Source: CAD feature listing. Evaluate the final solid. Frame: model axes, mm. Face numbers are marked on the shaded views. A direction names the side the tool comes from. Give positions to 0.01 mm unless a question says otherwise; leave off trailing zeros. Order: outer loops, then holes, each group sorted by start corner. A loop starts at its lowest first (then second) coordinate and runs counter-clockwise, first axis right, second up. Notation, with made-up numbers: (-1.5, 74.25) - (2.5, 74.25) arc R24 cw to (2.5, 92.25) - close; hole circle Ø7 at (9, 35). An arc over 180 degrees is marked (long way). Answer as CSV lines item,"result".
```python
from build123d import *

# Parameters (mm, degrees)
BOSS_EXTRUDE1_DEPTH = 30
SKETCH2_W           = 101
SKETCH2_H           = 2.2
CUT_EXTRUDE1_DEPTH  = 160
CUT_EXTRUDE2_DEPTH  = 108
CUT_EXTRUDE3_DEPTH  = 202
SKETCH6_W           = 165
SKETCH6_H           = 122.641754717
BOSS_EXTRUDE2_DEPTH = 2
SKETCH7_R           = 15
CUT_EXTRUDE4_DEPTH  = 22
CUT_EXTRUDE5_DEPTH  = 4.5
CUT_EXTRUDE6_DEPTH  = 21.5


with BuildPart() as part:
    # Sketch1 → Boss-Extrude1 (new body)
    with BuildSketch(Plane(origin=(0, 0, 0), x_dir=(1, 0, 0), z_dir=(0, 1, 0))):
        Polygon((-7.912176277, -15.186960462), (-7.912176277, 79.813039538), (148.087823723, 79.813039538), (148.087823723, 92.813039538), (-16.912176277, 92.813039538), (-16.912176277, -28.186960462), (148.087823723, -28.186960462), (148.087823723, -15.186960462), align=None)
    extrude(amount=BOSS_EXTRUDE1_DEPTH)

    # Sketch2 → Cut-Extrude1 (cut)
    with BuildSketch(Plane(origin=(148.087823723, 0, 0), x_dir=(0, 0, -1), z_dir=(1, 0, 0))):
        with Locations((32.313039538, 6.1)):
            Rectangle(SKETCH2_W, SKETCH2_H)
    extrude(amount=-CUT_EXTRUDE1_DEPTH, mode=Mode.SUBTRACT)

    # Sketch4 → Cut-Extrude2 (cut)
    with BuildSketch(Plane.XZ.offset(-7.2)):
        Polygon((-7.912176277, 15.186960462), (-11.910877917, 15.186960462), (-11.910877917, -79.815923725), (-7.912176277, -79.813039538), align=None)
    extrude(amount=CUT_EXTRUDE2_DEPTH, mode=Mode.SUBTRACT)

    # Sketch5 → Cut-Extrude3 (cut)
    with BuildSketch(Plane.ZY.offset(16.912176277)):
        Polygon((-92.813039538, 10), (-92.813039538, 30), (28.186960462, 30), align=None)
    extrude(amount=-CUT_EXTRUDE3_DEPTH, mode=Mode.SUBTRACT)

    # Sketch6 → Boss-Extrude2 (add)
    with BuildSketch(Plane(origin=(0, 24.667080359, -4.077203365), x_dir=(1, 0, 0), z_dir=(0, 0.986613411390535, -0.16307659692405538))):
        with Locations((65.587823723, 28.618946233)):
            Rectangle(SKETCH6_W, SKETCH6_H)
    extrude(amount=BOSS_EXTRUDE2_DEPTH)

    # Sketch7 → Cut-Extrude4 (cut)
    with BuildSketch(Plane.XY.offset(28.186960462)):
        with Locations((148.087823723, 0)):
            Circle(SKETCH7_R)
    extrude(amount=-CUT_EXTRUDE4_DEPTH, mode=Mode.SUBTRACT)

    # Sketch8 → Cut-Extrude5 (cut)
    with BuildSketch(Plane(origin=(148.087823723, 0, 0), x_dir=(0, 0, -1), z_dir=(1, 0, 0))):
        Polygon((-28.186960462, 30), (-28.186960462, 0), (92.813039538, 0), (92.813039538, 10), (93.139192732, 11.973226823), (-27.860807268, 31.973226823), align=None)
    extrude(amount=-CUT_EXTRUDE5_DEPTH, mode=Mode.SUBTRACT)

    # Sketch9 → Cut-Extrude6 (cut)
    with BuildSketch(Plane.XY.offset(28.186960462)):
        with BuildLine():
            Line((133.087823723, 0), (143.587823723, 0))
            Line((143.587823723, 0), (143.587823723, 14.309088021))
            Line((143.587823723, 14.309088021), (143.587823723, 15))
            ThreePointArc((143.587823723, 15), (132.981222005, 10.606601718), (128.587823723, 0))
            Line((128.587823723, 0), (133.087823723, 0))
        make_face()
    extrude(amount=-CUT_EXTRUDE6_DEPTH, mode=Mode.SUBTRACT)


solid = part.part
```
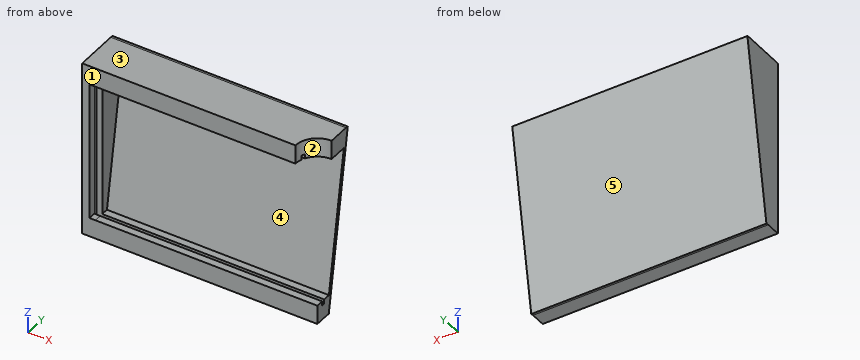
(1) Cut plane A-A (x = 91.5). Return loops of the section in (y, z).
Completed:
outline,"(0, -92.81) - (10, -92.81) - (11.97, -93.14) - (31.97, 27.86) - (30, 28.19) - (0, 28.19) - (0, 15.19) - (5, 15.19) - (5, 18.19) - (7.2, 18.19) - (7.2, 15.19) - (27.85, 15.19) - (12.15, -79.81) - (7.2, -79.81) - (7.2, -82.81) - (5, -82.81) - (5, -79.81) - (0, -79.81) - close"
(2) Mould query, pull axis Z, two halves, no side actions, for the marked faces 3, 4 and 5. Classes: released by +Z, released by -Z, zero draft, split by the parting line, or undercut.
Completed:
face 3,"released by +Z"
face 4,"undercut"
face 5,"released by -Z"
(3) Ray query, line 1 (Z direction, x = 99, y = 9); line 2 (X direction, y = 23.5, z = 2.5); line 3 (Y direction, x = 4, z = -82). Return the intervals inside material, ascending. Write a range as from..to.
Completed:
line 1,"-92.81..-79.81, 15.19..28.19"
line 2,"-16.91..-7.91"
line 3,"0..5, 7.2..13.81"
(4) Cut plane C-C (y = 24.5). Return loops of the section in (x, z), then the cut area to 3 significant figures.
Completed:
outline,"(-16.91, -17.35) - (143.59, -17.35) - (143.59, -5.09) - (-7.91, -5.09) - (-7.91, 15.19) - (143.59, 15.19) - (143.59, 28.19) - (-16.91, 28.19) - close"
area,"4,240 mm²"
(5) Access query for the marked faces 1 and 2. Directions: +Z, -Z, +X, -X, +Y, -Y. A direction counts if a zero-diameter tool reaches every point of the face in a straight line with its end or side. Return the directions, or none.
Completed:
face 1,"+Z, -Z, +X, -X, -Y"
face 2,"+Z, +X, -Y"
(6) Contact query for flat-ended pins moving along their axis: pin 1 (4 mm diameter, centred on x = 82.5, z = -1, fed in from +Y); pin 2 (1.5 mm diameter, centred on y = 3.5, z = -52, fed in from +X); pin 3 (11 mm diameter, centred on x = 100, y = 5, fed in from -Z); pin 4 (3 mm diameter, centred on y = 26.5, z = -20, fed in from -X). Output: stop coordinate, or through.
Completed:
pin 1,"y = 27.53"
pin 2,"x = -11.91"
pin 3,"z = -92.9"
pin 4,"through"
